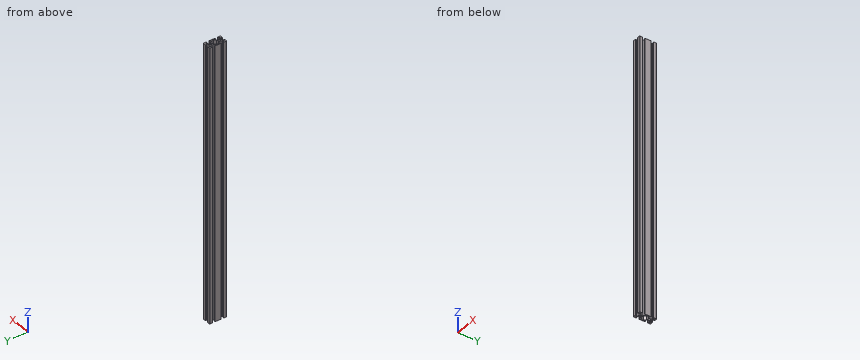
from build123d import *

# Parameters (mm, degrees)
SCHIZZO1_R                   = 2.1
ESTRUSIONE_ESTRUSIONE1_DEPTH = 650
RACCORDO1_R                  = 1


with BuildPart() as part:
    # Schizzo1 → Estrusione-Estrusione1 (new body)
    with BuildSketch(Plane.XY):
        Polygon((-3, 20), (-10, 20), (-10, 13), (-8, 13), (-8, 16), (-7, 16), (-4, 13), (-4, 7), (-7, 4), (-8, 4), (-8, 7), (-10, 7), (-10, -7), (-8, -7), (-8, -4), (-7, -4), (-4, -7), (-4, -13), (-7, -16), (-8, -16), (-8, -13), (-10, -13), (-10, -20), (-3, -20), (-3, -18), (-6, -18), (-6, -17), (-3, -14), (3, -14), (6, -17), (6, -18), (3, -18), (3, -20), (10, -20), (10, -13), (8, -13), (8, -16), (7, -16), (4, -13), (4, -7), (7, -4), (8, -4), (8, -7), (10, -7), (10, 7), (8, 7), (8, 4), (7, 4), (4, 7), (4, 13), (7, 16), (8, 16), (8, 13), (10, 13), (10, 20), (3, 20), (3, 18), (6, 18), (6, 17), (3, 14), (-3, 14), (-6, 17), (-6, 18), (-3, 18), align=None)
        Polygon((8, 2), (8, -2), (7, -2), (3, -6), (-3, -6), (-7, -2), (-8, -2), (-8, 2), (-7, 2), (-3, 6), (3, 6), (7, 2), align=None, mode=Mode.SUBTRACT)
        with Locations((0, 10)):
            Circle(SCHIZZO1_R, mode=Mode.SUBTRACT)
        with Locations((0, -10)):
            Circle(SCHIZZO1_R, mode=Mode.SUBTRACT)
    extrude(amount=ESTRUSIONE_ESTRUSIONE1_DEPTH)

    # Raccordo1
    raccordo1_edges = [part.edges().sort_by_distance(p)[0] for p in [
        (-10, 20, 325),
        (10, 20, 325),
        (10, -20, 325),
        (-10, -20, 325),
    ]]
    fillet(raccordo1_edges, radius=RACCORDO1_R)


solid = part.part
Geometry check sheet. Reference: the model listing, model coordinates, mm. Give positions to 0.01 mm unless a question says otherwise; leave off trailing zeros. One line per question, with ' | ' between items.
1. Gauge pin test, flat ends, axial feed: pin 1 (3 mm diameter, centred on x = 0.5, z = 402.5, fed in from -Y); pin 2 (1.8 mm diameter, centred on y = -11, z = 351, fed in from -X); pin 3 (1.8 mm diameter, centred on x = 0, z = 302, fed in from +Y). Record the tip position at first contact, or that the pin passes through.
Ans:
pin 1: y = -14 | pin 2: x = -4 | pin 3: y = 14
2. Scan lines: line 1 along Y through (x, z) = (0, 244.5); line 2 along Y through (x, z) = (4.5, 300); line 3 along Y through (x, z) = (4.75, 414.5). Record each from-to range of solid material in increasing order. Write a range as from..to.
Ans:
line 1: -14..-12.1, -7.9..-6, 6..7.9, 12.1..14 | line 2: -20..-18, -15.5..-13.5, -6.5..-4.5, 4.5..6.5, 13.5..15.5, 18..20 | line 3: -20..-18, -15.75..-13.75, -6.25..-4.25, 4.25..6.25, 13.75..15.75, 18..20
3. Cross-section at A-A (z = 43). Count the separate pieces of the cut face and the enclosed holes in it, plus the area to 3 significant figures.
Ans:
separate pieces: 1 | enclosed holes: 3 | area: 321 mm2
